from build123d import *

# Parameters (mm, degrees)
EXTRUDE_1_DEPTH          = 4.1
EXTRUDE_1_DEPTH_BACK     = 4.1
SKETCH_2_R               = 1
EXTRUDE_2_DEPTH          = 1.9
EXTRUDE_3_DEPTH          = 2
EXTRUDE_3_DEPTH_BACK     = 2
CUT_EXTRUDE_1_DEPTH      = 2
CUT_EXTRUDE_1_DEPTH_BACK = 2
FILLET_1_R               = 0.1


with BuildPart() as part:
    # Sketch 1 → Extrude 1 (new, two sides: drawn at the far end of the back side and taken through both)
    with BuildSketch(Plane.XY.offset(-EXTRUDE_1_DEPTH_BACK)):
        Polygon((-6, 0), (6, 0), (3.5, 1.7), (-3.5, 1.7), align=None)
    extrude(amount=EXTRUDE_1_DEPTH + EXTRUDE_1_DEPTH_BACK)

    # Sketch 2 → Extrude 2 (add)
    with BuildSketch(Plane.XY.offset(4.1)):
        with BuildLine():
            Line((0, 0), (-7.5, 0))
            Line((-7.5, 0), (-2.134627344, 8.801294011))
            ThreePointArc((-2.134627344, 8.801294011), (0, 10), (2.134627344, 8.801294011))
            Line((2.134627344, 8.801294011), (7.5, 0))
            Line((7.5, 0), (0, 0))
        make_face()
        with Locations(Location((0, 7.5, 0), (0, 0, 180))):
            Circle(SKETCH_2_R, mode=Mode.SUBTRACT)
    extrude_2 = extrude(amount=EXTRUDE_2_DEPTH)

    # Mirror 1: Extrude 2 across plane
    add(extrude_2.mirror(Plane.XY))

    # Sketch 3 → Extrude 3 (add, two sides: drawn at the far end of the back side and taken through both)
    with BuildSketch(Plane.XY.offset(-EXTRUDE_3_DEPTH_BACK)):
        with BuildLine():
            Line((1.5, 0), (-1.5, 0))
            Line((-1.5, 0), (-1.5, -0.677124344))
            ThreePointArc((-1.5, -0.677124344), (-1.780042303, -1.088161527), (-1.95, -1.555590279))
            Line((-1.95, -1.555590279), (-1.95, -2.5))
            Line((-1.95, -2.5), (1.95, -2.5))
            Line((1.95, -2.5), (1.95, -1.555590279))
            ThreePointArc((1.95, -1.555590279), (1.780042303, -1.088161527), (1.5, -0.677124344))
            Line((1.5, -0.677124344), (1.5, 0))
        make_face()
    extrude(amount=EXTRUDE_3_DEPTH + EXTRUDE_3_DEPTH_BACK)

    # Sketch 4 → Cut-Extrude 1 (cut, two sides: drawn at the far end of the back side and taken through both)
    with BuildSketch(Plane(origin=(0, 0, 0), x_dir=(0, 0, -1), z_dir=(1, 0, 0)).offset(-CUT_EXTRUDE_1_DEPTH_BACK)):
        with BuildLine():
            Line((-1.5, 0), (-1.5, -0.677124344))
            ThreePointArc((-1.5, -0.677124344), (-1.780042303, -1.088161527), (-1.95, -1.555590279))
            Line((-1.95, -1.555590279), (-1.95, -2.5))
            Line((-1.95, -2.5), (-2, -2.5))
            Line((-2, -2.5), (-2, 0))
            Line((-2, 0), (-1.5, 0))
        make_face()
        with BuildLine():
            Line((2, 0), (1.5, 0))
            Line((1.5, 0), (1.5, -0.677124344))
            ThreePointArc((1.5, -0.677124344), (1.780042303, -1.088161527), (1.95, -1.555590279))
            Line((1.95, -1.555590279), (1.95, -2.5))
            Line((1.95, -2.5), (2, -2.5))
            Line((2, -2.5), (2, 0))
        make_face()
    extrude(amount=CUT_EXTRUDE_1_DEPTH + CUT_EXTRUDE_1_DEPTH_BACK, mode=Mode.SUBTRACT)

    # Fillet 1
    fillet_1_edges = [part.edges().sort_by_distance(p)[0] for p in [
        (0, -2.5, 1.95),
        (-1.95, -2.5, 0),
        (1.95, -2.5, 0),
        (0, -2.5, -1.95),
    ]]
    fillet(fillet_1_edges, radius=FILLET_1_R)


solid = part.part
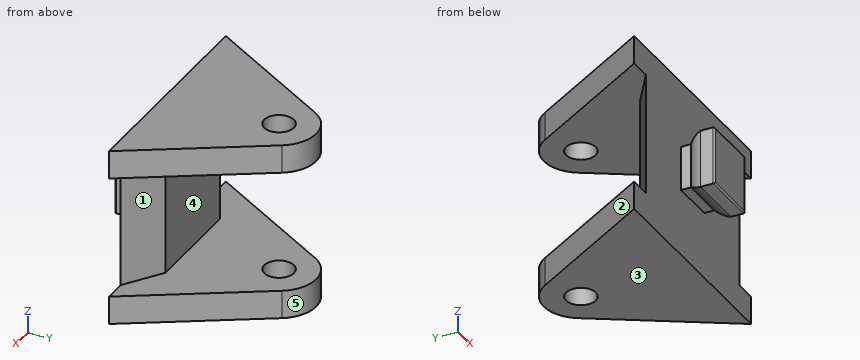
The listing builds one solid part. Answer for the finished solid, in the listing's coordinates (mm). Face numbers are marked on the shaded views. A direction names the side the tool comes from. Coordinates: 2 decimals unless noted, no trailing zeros. Write each loop counter-clockwise with the first axis right and the second up, starting at its lowest first coordinate (ties: lowest second). Pieces come first, ordered by that corner, then holes. Notation, with made-up numbers: M 36.25,20 L 90.25,20 A11 cw 90.25,28 Z; hole C 5.25,68 d11. An arc over 180 degrees is marked long. Use one line per item in the form item = value.
Item 1: Find section B-B, the plane z = 5. Give the vertices of the cut face in (x, y), plus the area to 3 significant figures.
Model answer:
outline = M -7.5,0 L 7.5,0 L 2.13,8.8 A2.5 ccw -2.13,8.8 Z; hole C 0,7.5 d2
area = 85.3 mm2
Item 2: Find section C-C, the plane y = 7.5. Give the vertices of the cut face in (x, z), plus the area to 3 significant figures.
Model answer:
outline = M -2.93,-6 L -1,-6 L -1,-4.1 L -2.93,-4.1 Z; M -2.93,4.1 L -1,4.1 L -1,6 L -2.93,6 Z; M 1,-6 L 2.93,-6 L 2.93,-4.1 L 1,-4.1 Z; M 1,4.1 L 2.93,4.1 L 2.93,6 L 1,6 Z
area = 14.7 mm2
Item 3: Find section A-A, the plane x = 0. Give the vertices of the cut face in (y, z).
Model answer:
outline = M -2.5,-1.85 A0.1 ccw -2.4,-1.95 L -1.56,-1.95 A2 ccw -0.68,-1.5 L 0,-1.5 L 0,-6 L 6.5,-6 L 6.5,-4.1 L 1.7,-4.1 L 1.7,4.1 L 6.5,4.1 L 6.5,6 L 0,6 L 0,1.5 L -0.68,1.5 A2 ccw -1.56,1.95 L -2.4,1.95 A0.1 ccw -2.5,1.85 Z; M 8.5,-6 L 10,-6 L 10,-4.1 L 8.5,-4.1 Z; M 8.5,4.1 L 10,4.1 L 10,6 L 8.5,6 Z
Item 4: Find section D-D, the plane y = 2.75. Give the vertices of the cut face in (x, z), plus the area to 3 significant figures.
Model answer:
outline = M -5.82,-6 L 5.82,-6 L 5.82,-4.1 L -5.82,-4.1 Z; M -5.82,4.1 L 5.82,4.1 L 5.82,6 L -5.82,6 Z
area = 44.3 mm2
Item 5: Given P1, Ø2.5, axis at x = 0, y = 7.5, coming from the -Z side; P2, Ø1.2, axis at x = 0, y = 7.5, coming from the +Z side; P3, Ø0.7, axis at x = 0.5, y = -2, coming from the -Z side; P4, Ø0.7, axis at y = -2, z = 1, coming from the -X side, each flat-ended and moving along its own axis, determine where each tip first touches the part or whether it passes through.
Model answer:
P1 = -6
P2 = through
P3 = -1.95
P4 = -1.95
Item 6: For the marked faces 1 and 2, determine the directions among +Z, -Z, +X, -X, +Y, -Y from which every point of the face is accessible in a straight line to the end or side of a thin tool.
Model answer:
face_1 = +X, +Y
face_2 = +Z, -Z, -X, +Y
Item 7: The mould has two halves that part along Z. Classify the marked faces 3, 4 and 5: released by +Z, released by -Z, zero draft, split by the parting line, or undercut.
Model answer:
face_3 = released by -Z
face_4 = undercut
face_5 = zero draft
Item 8: Find the intervals of material crossed by probe 1 along Z at (x, y) = (0.5, 6.5); probe 2 along Y at (x, z) = (0, -4.5); probe 3 along X at (y, z) = (7.5, 4.95), in increasing order.
Model answer:
probe_1 = -6 to -4.1, 4.1 to 6
probe_2 = 0 to 6.5, 8.5 to 10
probe_3 = -2.93 to -1, 1 to 2.93
